Verification items for the finished model (mm, model axes). Coordinates: 2 decimals unless noted, no trailing zeros. Order: outer loops, then holes, each group sorted by start corner. A loop starts at its lowest first (then second) coordinate and runs counter-clockwise, first axis right, second up. Notation, with made-up numbers: M -27.75,47 L -6.75,47 A32 ccw -6.75,75 Z; hole C 15.25,-20.5 d8. An arc over 180 degrees is marked long. Return JSON: item names as keys, results as strings. Group by question number.
Q1. Section check A-A, the plane x = 8.75. Enter the section's corners in (y, z).
Q2. Go/stop test with a flat-tipped pin: pin 1 Ø4 at (x, y) = (4.5, 216) entering from +Z. Record where the tip stops, or that it passes through.
Q3. Section check D-D, the plane z = 215. Enter the section's corners in (x, y), then the cut area to 3 significant figures.
Q4. Section check C-C, the plane y = 269. Enter the section's corners in (x, z).
Q5. Section check B-B, the plane z = 118.5. Enter the section's corners in (x, y), then the cut area to 3 significant figures.
Q6. Thickness scan on probe 1 along Y at (x, z) = (5, 304); probe 2 along Z at (x, y) = (10.5, 277); probe 3 along Y at (x, z) = (1.5, 285.5). Record the ranges inside material, lowest first.
from build123d import *

# Parameters (mm, degrees)
F0_W     = 101.6
F0_H     = 19.05
F1_DEPTH = 17.78


# Not quite as in the source:
# - a feature names something its author has since deleted; it is built from what else it names


with BuildPart() as f1:
    # F0 (on Right) → F1 (new body)
    with BuildSketch(Plane.YZ):
        with BuildLine():
            ThreePointArc((508, 457.2), (375.1962383216, 406.7634952275), (254, 332.6544408126))
            Line((254, 332.6544408126), (254, 0))
            Line((254, 0), (330.2, 0))
            Line((330.2, 0), (431.8, 0))
            Line((431.8, 0), (508, 0))
            Line((508, 0), (508, 457.2))
        make_face()
        Polygon((349.8489306504, 132.4179212181), (367.2235539314, 180.154306354), (383.9312887289, 174.0731882056), (349.182042167, 78.6004179338), (332.4743073695, 84.6815360821), align=None, mode=Mode.SUBTRACT)
        Polygon((401.9728004932, 275.6270766258), (419.3474237742, 323.3634617617), (436.7220470551, 371.0998468977), (453.4297818527, 365.0187287493), (418.6805352908, 269.5459584775), align=None, mode=Mode.SUBTRACT)
        Polygon((127, 0), (76.2, 0), (76.2, -19.05), (177.8, -19.05), (177.8, 0), align=None)
        with BuildLine():
            ThreePointArc((254, 332.6544408126), (103.8213611206, 184.0253886947), (0, 0))
            Line((0, 0), (76.2, 0))
            Line((76.2, 0), (127, 0))
            Line((127, 0), (177.8, 0))
            Line((177.8, 0), (254, 0))
            Line((254, 0), (254, 332.6544408126))
        make_face()
        with Locations((381, -9.525)):
            Rectangle(F0_W, F0_H)
    extrude(amount=F1_DEPTH)


solid = f1.part
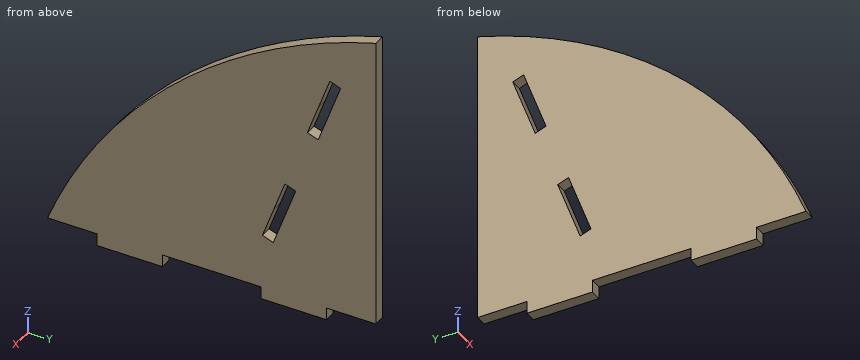
Numbers:
{
 "1": {"outline": "M 0,0 L 76.2,0 L 76.2,-19.05 L 177.8,-19.05 L 177.8,0 L 330.2,0 L 330.2,-19.05 L 431.8,-19.05 L 431.8,0 L 508,0 L 508,457.2 A765.43 ccw Z; hole M 332.47,84.68 L 349.18,78.6 L 383.93,174.07 L 367.22,180.15 Z; hole M 401.97,275.63 L 418.68,269.55 L 453.43,365.02 L 436.72,371.1 Z"},
 "2": {"pin 1": "stops at z = 304.03"},
 "3": {"outline": "M 0,128.77 L 17.78,128.77 L 17.78,508 L 0,508 Z", "area": "6,740 mm2"},
 "4": {"outline": "M 0,0 L 17.78,0 L 17.78,343.58 L 0,343.58 Z"},
 "5": {"outline": "M 0,58.97 L 17.78,58.97 L 17.78,344.78 L 0,344.78 Z; M 0,363.7 L 17.78,363.7 L 17.78,508 L 0,508 Z", "area": "7,650 mm2"},
 "6": {"probe 1": "y = 217.97 to 412.3, 431.22 to 508", "probe 2": "z = 0 to 349.19", "probe 3": "y = 196.88 to 405.57, 424.49 to 508"}
}
